```python
from build123d import *

# Parameters (mm, degrees)
CROQUIS1_R              = 10
CROQUIS1_R_2            = 3
SALIENTE_EXTRUIR1_DEPTH = 19
CROQUIS2_R              = 10
SALIENTE_EXTRUIR2_DEPTH = 19
CROQUIS3_R              = 10
CORTAR_EXTRUIR1_DEPTH   = 20
CROQUIS4_R              = 12.5
CORTAR_EXTRUIR2_DEPTH   = 2
CROQUIS5_R              = 12.5
CORTAR_EXTRUIR3_DEPTH   = 2


with BuildPart() as part:
    # Croquis1 → Saliente-Extruir1 (new body)
    with BuildSketch(Plane(origin=(0, 0, 0), x_dir=(1, 0, 0), z_dir=(0, 1, 0))):
        Circle(CROQUIS1_R)
        Circle(CROQUIS1_R_2, mode=Mode.SUBTRACT)
    extrude(amount=SALIENTE_EXTRUIR1_DEPTH)

    # Croquis2 → Saliente-Extruir2 (add)
    with BuildSketch(Plane(origin=(0, 19, 0), x_dir=(1, 0, 0), z_dir=(0, 1, 0))):
        with BuildLine():
            Line((-1.5, -19.943670675), (0, -24))
            Line((0, -24), (1.5, -19.943670675))
            ThreePointArc((1.5, -19.943670675), (1.569181915, -19.938346675), (1.638344942, -19.932782692))
            Line((1.638344942, -19.932782692), (3.754427161, -23.704520174))
            Line((3.754427161, -23.704520174), (4.601409964, -19.463479297))
            ThreePointArc((4.601409964, -19.463479297), (4.668907277, -19.447398408), (4.736348394, -19.431083446))
            Line((4.736348394, -19.431083446), (7.416407865, -22.825356391))
            Line((7.416407865, -22.825356391), (7.589517943, -18.504032463))
            ThreePointArc((7.589517943, -18.504032463), (7.653668647, -18.47759065), (7.71772723, -18.450926437))
            Line((7.71772723, -18.450926437), (10.895771994, -21.384156581))
            Line((10.895771994, -21.384156581), (10.390746803, -17.088954938))
            ThreePointArc((10.390746803, -17.088954938), (10.449971294, -17.052803287), (10.509070008, -17.016446385))
            Line((10.509070008, -17.016446385), (14.106846055, -19.416407865))
            Line((14.106846055, -19.416407865), (12.936120991, -15.253090628))
            ThreePointArc((12.936120991, -15.253090628), (12.988960967, -15.208119312), (13.041644604, -15.162964948))
            Line((13.041644604, -15.162964948), (16.970562748, -16.970562748))
            Line((16.970562748, -16.970562748), (15.162964948, -13.041644604))
            ThreePointArc((15.162964948, -13.041644604), (15.208119312, -12.988960967), (15.253090628, -12.936120991))
            Line((15.253090628, -12.936120991), (19.416407865, -14.106846055))
            Line((19.416407865, -14.106846055), (17.016446385, -10.509070008))
            ThreePointArc((17.016446385, -10.509070008), (17.052803287, -10.449971294), (17.088954938, -10.390746803))
            Line((17.088954938, -10.390746803), (21.384156581, -10.895771994))
            Line((21.384156581, -10.895771994), (18.450926437, -7.71772723))
            ThreePointArc((18.450926437, -7.71772723), (18.47759065, -7.653668647), (18.504032463, -7.589517943))
            Line((18.504032463, -7.589517943), (22.825356391, -7.416407865))
            Line((22.825356391, -7.416407865), (19.431083446, -4.736348394))
            ThreePointArc((19.431083446, -4.736348394), (19.447398408, -4.668907277), (19.463479297, -4.601409964))
            Line((19.463479297, -4.601409964), (23.704520174, -3.754427161))
            Line((23.704520174, -3.754427161), (19.932782692, -1.638344942))
            ThreePointArc((19.932782692, -1.638344942), (19.938346675, -1.569181915), (19.943670675, -1.5))
            Line((19.943670675, -1.5), (24, 0))
            Line((24, 0), (19.943670675, 1.5))
            ThreePointArc((19.943670675, 1.5), (19.938346675, 1.569181915), (19.932782692, 1.638344942))
            Line((19.932782692, 1.638344942), (23.704520174, 3.754427161))
            Line((23.704520174, 3.754427161), (19.463479297, 4.601409964))
            ThreePointArc((19.463479297, 4.601409964), (19.447398408, 4.668907277), (19.431083446, 4.736348394))
            Line((19.431083446, 4.736348394), (22.825356391, 7.416407865))
            Line((22.825356391, 7.416407865), (18.504032463, 7.589517943))
            ThreePointArc((18.504032463, 7.589517943), (18.47759065, 7.653668647), (18.450926437, 7.71772723))
            Line((18.450926437, 7.71772723), (21.384156581, 10.895771994))
            Line((21.384156581, 10.895771994), (17.088954938, 10.390746803))
            ThreePointArc((17.088954938, 10.390746803), (17.052803287, 10.449971294), (17.016446385, 10.509070008))
            Line((17.016446385, 10.509070008), (19.416407865, 14.106846055))
            Line((19.416407865, 14.106846055), (15.253090628, 12.936120991))
            ThreePointArc((15.253090628, 12.936120991), (15.208119312, 12.988960967), (15.162964948, 13.041644604))
            Line((15.162964948, 13.041644604), (16.970562748, 16.970562748))
            Line((16.970562748, 16.970562748), (13.041644604, 15.162964948))
            ThreePointArc((13.041644604, 15.162964948), (12.988960967, 15.208119312), (12.936120991, 15.253090628))
            Line((12.936120991, 15.253090628), (14.106846055, 19.416407865))
            Line((14.106846055, 19.416407865), (10.509070008, 17.016446385))
            ThreePointArc((10.509070008, 17.016446385), (10.449971294, 17.052803287), (10.390746803, 17.088954938))
            Line((10.390746803, 17.088954938), (10.895771994, 21.384156581))
            Line((10.895771994, 21.384156581), (7.71772723, 18.450926437))
            ThreePointArc((7.71772723, 18.450926437), (7.653668647, 18.47759065), (7.589517943, 18.504032463))
            Line((7.589517943, 18.504032463), (7.416407865, 22.825356391))
            Line((7.416407865, 22.825356391), (4.736348394, 19.431083446))
            ThreePointArc((4.736348394, 19.431083446), (4.668907277, 19.447398408), (4.601409964, 19.463479297))
            Line((4.601409964, 19.463479297), (3.754427161, 23.704520174))
            Line((3.754427161, 23.704520174), (1.638344942, 19.932782692))
            ThreePointArc((1.638344942, 19.932782692), (1.569181915, 19.938346675), (1.5, 19.943670675))
            Line((1.5, 19.943670675), (0, 24))
            Line((0, 24), (-1.5, 19.943670675))
            ThreePointArc((-1.5, 19.943670675), (-1.569181915, 19.938346675), (-1.638344942, 19.932782692))
            Line((-1.638344942, 19.932782692), (-3.754427161, 23.704520174))
            Line((-3.754427161, 23.704520174), (-4.601409964, 19.463479297))
            ThreePointArc((-4.601409964, 19.463479297), (-4.668907277, 19.447398408), (-4.736348394, 19.431083446))
            Line((-4.736348394, 19.431083446), (-7.416407865, 22.825356391))
            Line((-7.416407865, 22.825356391), (-7.589517943, 18.504032463))
            ThreePointArc((-7.589517943, 18.504032463), (-7.653668647, 18.47759065), (-7.71772723, 18.450926437))
            Line((-7.71772723, 18.450926437), (-10.895771994, 21.384156581))
            Line((-10.895771994, 21.384156581), (-10.390746803, 17.088954938))
            ThreePointArc((-10.390746803, 17.088954938), (-10.449971294, 17.052803287), (-10.509070008, 17.016446385))
            Line((-10.509070008, 17.016446385), (-14.106846055, 19.416407865))
            Line((-14.106846055, 19.416407865), (-12.936120991, 15.253090628))
            ThreePointArc((-12.936120991, 15.253090628), (-12.988960967, 15.208119312), (-13.041644604, 15.162964948))
            Line((-13.041644604, 15.162964948), (-16.970562748, 16.970562748))
            Line((-16.970562748, 16.970562748), (-15.162964948, 13.041644604))
            ThreePointArc((-15.162964948, 13.041644604), (-15.208119312, 12.988960967), (-15.253090628, 12.936120991))
            Line((-15.253090628, 12.936120991), (-19.416407865, 14.106846055))
            Line((-19.416407865, 14.106846055), (-17.016446385, 10.509070008))
            ThreePointArc((-17.016446385, 10.509070008), (-17.052803287, 10.449971294), (-17.088954938, 10.390746803))
            Line((-17.088954938, 10.390746803), (-21.384156581, 10.895771994))
            Line((-21.384156581, 10.895771994), (-18.450926437, 7.71772723))
            ThreePointArc((-18.450926437, 7.71772723), (-18.47759065, 7.653668647), (-18.504032463, 7.589517943))
            Line((-18.504032463, 7.589517943), (-22.825356391, 7.416407865))
            Line((-22.825356391, 7.416407865), (-19.431083446, 4.736348394))
            ThreePointArc((-19.431083446, 4.736348394), (-19.447398408, 4.668907277), (-19.463479297, 4.601409964))
            Line((-19.463479297, 4.601409964), (-23.704520174, 3.754427161))
            Line((-23.704520174, 3.754427161), (-19.932782692, 1.638344942))
            ThreePointArc((-19.932782692, 1.638344942), (-19.938346675, 1.569181915), (-19.943670675, 1.5))
            Line((-19.943670675, 1.5), (-24, 0))
            Line((-24, 0), (-19.943670675, -1.5))
            ThreePointArc((-19.943670675, -1.5), (-19.938346675, -1.569181915), (-19.932782692, -1.638344942))
            Line((-19.932782692, -1.638344942), (-23.704520174, -3.754427161))
            Line((-23.704520174, -3.754427161), (-19.463479297, -4.601409964))
            ThreePointArc((-19.463479297, -4.601409964), (-19.447398408, -4.668907277), (-19.431083446, -4.736348394))
            Line((-19.431083446, -4.736348394), (-22.825356391, -7.416407865))
            Line((-22.825356391, -7.416407865), (-18.504032463, -7.589517943))
            ThreePointArc((-18.504032463, -7.589517943), (-18.47759065, -7.653668647), (-18.450926437, -7.71772723))
            Line((-18.450926437, -7.71772723), (-21.384156581, -10.895771994))
            Line((-21.384156581, -10.895771994), (-17.088954938, -10.390746803))
            ThreePointArc((-17.088954938, -10.390746803), (-17.052803287, -10.449971294), (-17.016446385, -10.509070008))
            Line((-17.016446385, -10.509070008), (-19.416407865, -14.106846055))
            Line((-19.416407865, -14.106846055), (-15.253090628, -12.936120991))
            ThreePointArc((-15.253090628, -12.936120991), (-15.208119312, -12.988960967), (-15.162964948, -13.041644604))
            Line((-15.162964948, -13.041644604), (-16.970562748, -16.970562748))
            Line((-16.970562748, -16.970562748), (-13.041644604, -15.162964948))
            ThreePointArc((-13.041644604, -15.162964948), (-12.988960967, -15.208119312), (-12.936120991, -15.253090628))
            Line((-12.936120991, -15.253090628), (-14.106846055, -19.416407865))
            Line((-14.106846055, -19.416407865), (-10.509070008, -17.016446385))
            ThreePointArc((-10.509070008, -17.016446385), (-10.449971294, -17.052803287), (-10.390746803, -17.088954938))
            Line((-10.390746803, -17.088954938), (-10.895771994, -21.384156581))
            Line((-10.895771994, -21.384156581), (-7.71772723, -18.450926437))
            ThreePointArc((-7.71772723, -18.450926437), (-7.653668647, -18.47759065), (-7.589517943, -18.504032463))
            Line((-7.589517943, -18.504032463), (-7.416407865, -22.825356391))
            Line((-7.416407865, -22.825356391), (-4.736348394, -19.431083446))
            ThreePointArc((-4.736348394, -19.431083446), (-4.668907277, -19.447398408), (-4.601409964, -19.463479297))
            Line((-4.601409964, -19.463479297), (-3.754427161, -23.704520174))
            Line((-3.754427161, -23.704520174), (-1.638344942, -19.932782692))
            ThreePointArc((-1.638344942, -19.932782692), (-1.569181915, -19.938346675), (-1.5, -19.943670675))
        make_face()
        Circle(CROQUIS2_R, mode=Mode.SUBTRACT)
    extrude(amount=-SALIENTE_EXTRUIR2_DEPTH)

    # Croquis3 → Cortar-Extruir1 (cut, through all)
    with BuildSketch(Plane.XZ):
        Circle(CROQUIS3_R)
    extrude(amount=-CORTAR_EXTRUIR1_DEPTH, mode=Mode.SUBTRACT)

    # Croquis4 → Cortar-Extruir2 (cut)
    with BuildSketch(Plane(origin=(0, 19, 0), x_dir=(1, 0, 0), z_dir=(0, 1, 0))):
        Circle(CROQUIS4_R)
    extrude(amount=-CORTAR_EXTRUIR2_DEPTH, mode=Mode.SUBTRACT)

    # Croquis5 → Cortar-Extruir3 (cut)
    with BuildSketch(Plane.XZ):
        Circle(CROQUIS5_R)
    extrude(amount=-CORTAR_EXTRUIR3_DEPTH, mode=Mode.SUBTRACT)


solid = part.part
```
Geometry check sheet. Reference: the model listing, model coordinates, mm. A direction names the side the tool comes from. Give positions to 0.01 mm unless a question says otherwise; leave off trailing zeros. Order: outer loops, then holes, each group sorted by start corner. A loop starts at its lowest first (then second) coordinate and runs counter-clockwise, first axis right, second up.
1. Gauge pin test, flat ends, axial feed: pin 1 Ø12 at (x, z) = (-1, -4) entering from +Y; pin 2 Ø10 at (y, z) = (10.5, 15.5) entering from -X; pin 3 Ø16 at (x, z) = (0, 0) entering from +Y. Record the tip position at first contact, or that the pin passes through.
2. Release check for a two-part mould opening along Z. For faces 4 (the face through (21.614, 9.633, -4.172)), 5 (the face through (-9.33, 9.63, 19.94)), 6 (the face through (2.711, 9.633, -21.845)) record: pulls with the +Z half, pulls with the -Z half, needs draft (parallel to the pull), parting line crosses it, or undercut.
3. Thickness scan on L1, parallel to X at y = 4, z = 21.5; L2, parallel to X at y = 18.25, z = 16; L3, parallel to Z at x = -19, y = 15.25. Record the ranges inside material, lowest first.
4. Access from +Z, -Z, +X, -X, +Y, -Y to the whole of each face (thin tool, end or side, straight path). Record for faces 1 (the face through (0.74, 9.63, 22)), 2 (the face through (-10.64, 9.63, 19.21)), 3 (the face through (-6.058, 9.633, -21.104)).
5. Section check A-A, the plane x = 6. Enter the section's corners in (y, z).
6. Section check B-B, the plane x = -5.5. Enter the section's corners in (y, z).
Values follow:
1. pin 1: stops at y = 17
1. pin 2: stops at x = -21.38
1. pin 3: passes through
2. face 4: undercut
2. face 5: pulls with the +Z half
2. face 6: pulls with the -Z half
3. L1: x = -7.47 to -6.37, -4.19 to -2.52, -0.92 to 0.92, 2.52 to 4.19, 6.37 to 7.47
3. L2: x = -16.52 to -14.86, -13.15 to 13.15, 14.86 to 16.52
3. L3: z = -13.99 to -13.48, -10.62 to -8.31, -7.57 to 7.57, 8.31 to 10.62, 13.48 to 13.99
4. face 1: +Z, +Y, -Y
4. face 2: +Y, -Y
4. face 3: -Z, +Y, -Y
5. outline: (0, -21.03) - (19, -21.03) - (19, -10.97) - (17, -10.97) - (17, -8) - (2, -8) - (2, -10.97) - (0, -10.97) - close; (0, 10.97) - (2, 10.97) - (2, 8) - (17, 8) - (17, 10.97) - (19, 10.97) - (19, 21.03) - (0, 21.03) - close
6. outline: (0, -20.4) - (19, -20.4) - (19, -11.22) - (17, -11.22) - (17, -8.35) - (2, -8.35) - (2, -11.22) - (0, -11.22) - close; (0, 11.22) - (2, 11.22) - (2, 8.35) - (17, 8.35) - (17, 11.22) - (19, 11.22) - (19, 20.4) - (0, 20.4) - close
